Autodesk Inventor part; units mm, degrees
ref_plane "YZ Plane" through (0, 0, 0) normal (1, 0, 0) x (0, 1, 0)
ref_plane "XZ Plane" through (0, 0, 0) normal (0, 1, 0) x (-1, 0, 0)
ref_plane "XY Plane" through (0, 0, 0) normal (0, 0, 1) x (1, 0, 0)
sketch "Sketch1" plane through (0, 0, 0) normal (1, 0, 0) x (0, 1, 0)
  line L0 (7.987, -6.35) -> (11, -6.35)
  line L1 (11, -6.35) -> (11, -4.75)
  line L2 (11, -4.75) -> (8.75, -4.75)
  line L3 (8.75, -4.75) -> (8.75, 4.75)
  line L4 (8.75, 4.75) -> (11, 4.75)
  line L5 (11, 4.75) -> (11, 6.35)
  line L6 (11, 6.35) -> (7.987, 6.35)
  line L7 (7.987, 6.35) -> (7.987, 1.55)
  line L8 (7.987, 1.55) -> (6.945, 1.55)
  line L9 (6.945, 1.55) -> (6.945, -1.55)
  line L10 (6.945, -1.55) -> (7.987, -1.55)
  line L11 (7.987, -1.55) -> (7.987, -6.35)
  line L12 (0, 0) -> (0, 23.3621) construction
  line L13 (6.945, 0) -> (8.75, 0) construction
  dimension "d0" = 9.5
  dimension "d1" = 15.974
  dimension "d2" = 13.89
  dimension "d3" = 3.1
  dimension "d4" = 12.7
  dimension "d5" = 17.5
  dimension "d6" = 22
revolve "Revolution1" add sketch "Sketch1" angle 360 about axis through (0, 0, 0) along (0, 0, 1)
chamfer "Chamfer1" distance 0.3 angle 45 2 edges at (0, -7.987, 6.35) (0, -7.987, -6.35)
ref_plane "Work Plane1" through (0, 0, 0) normal (0, 0, -1) x (-1, 0, 0)
properties part number "idler pulley" material "ABS Plastic"
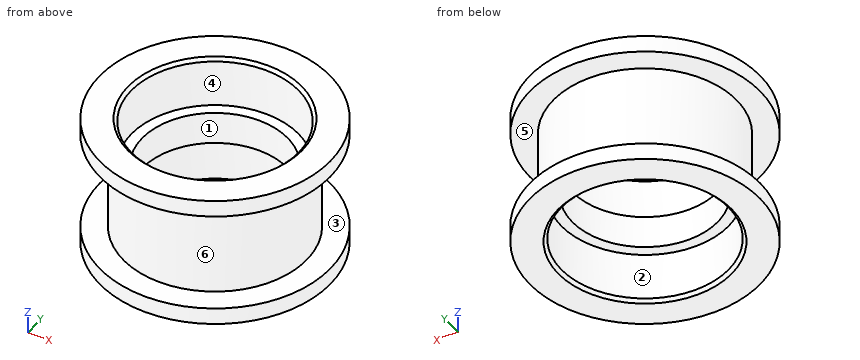
Source: CAD feature listing. Evaluate the final solid. Frame: model axes, mm. Face numbers are marked on the shaded views. A direction names the side the tool comes from. Give positions to 0.01 mm unless a question says otherwise; leave off trailing zeros. Loops run counter-clockwise (first coordinate to the right, second up) from the corner with the lowest first, then second, coordinate; pieces in that order, holes last. Notation, with made-up numbers: (65, -10) -> (75, -10) arc R25 ccw to (75, 13) -> close; hole circle Ø3 at (51, 10). An arc over 180 degrees is marked (long way). Use a Markdown table: item, result. Add a question column.
(1) Section query C-C (z = -3.5). Output: boundary loops of the cut face in (x, y), then the cut area to 3 significant figures.
(2) Section query A-A (x = 0). Output: boundary loops of the cut face in (y, z) (3 decimals), then the cut area to 3 significant figures.
(3) First-contact query: pin 1 Ø3 at (x, z) = (-4.5, 2) entering from -Y; pin 2 Ø13 at (x, y) = (0.5, -0.5) entering from -Z; pin 3 Ø4 at (x, z) = (-2, 3) entering from -Y. Flat tips, straight axial feed; report the tip coordinate or a pass-through.
(4) Pull-direction query (X, two-part tool) for the marked faces 4, 5 and 6; classes: +X half, -X half, draft (parallel to the pull), parting line (faces both ways), or undercut.
(5) Section query D-D (z = -1.25). Output: boundary loops of the cut face in (x, y) (3 decimals), then the cut area to 3 significant figures.
(6) Ray query, line 1 (Z direction, x = -9, y = -2.75); line 2 (Y direction, x = 0, z = -0.6) (3 decimals); line 3 (X direction, y = 0, z = -4.95). Return the intervals inside material, ascending.
(7) Access query for the marked faces 1, 2 and 3. Directions: +Z, -Z, +X, -X, +Y, -Y. A direction counts if a zero-diameter tool reaches every point of the face in a straight line with its end or side. Return the directions, or none.
Checked values:
| question | item | result |
|---|---|---|
| 1 | outline | circle Ø17.5 at (0, 0); hole circle Ø15.97 at (0, 0) |
| 1 | area | 40.1 mm^2 |
| 2 | outline | (-11, -6.35) -> (-8.287, -6.35) -> (-7.987, -6.05) -> (-7.987, -1.55) -> (-6.945, -1.55) -> (-6.945, 1.55) -> (-7.987, 1.55) -> (-7.987, 6.05) -> (-8.287, 6.35) -> (-11, 6.35) -> (-11, 4.75) -> (-8.75, 4.75) -> (-8.75, -4.75) -> (-11, -4.75) -> close; (6.945, -1.55) -> (7.987, -1.55) -> (7.987, -6.05) -> (8.287, -6.35) -> (11, -6.35) -> (11, -4.75) -> (8.75, -4.75) -> (8.75, 4.75) -> (11, 4.75) -> (11, 6.35) -> (8.287, 6.35) -> (7.987, 6.05) -> (7.987, 1.55) -> (6.945, 1.55) -> close |
| 2 | area | 40.1 mm^2 |
| 3 | pin 1 | y = -8.22 |
| 3 | pin 2 | z = -1.55 |
| 3 | pin 3 | y = -10.95 |
| 4 | face 4 | undercut |
| 4 | face 5 | draft |
| 4 | face 6 | parting line |
| 5 | outline | circle Ø17.5 at (0, 0); hole circle Ø13.89 at (0, 0) |
| 5 | area | 89.0 mm^2 |
| 6 | line 1 | -6.35 to -4.75, 4.75 to 6.35 |
| 6 | line 2 | -8.75 to -6.945, 6.945 to 8.75 |
| 6 | line 3 | -11 to -7.99, 7.99 to 11 |
| 7 | face 1 | +Z, -Z |
| 7 | face 2 | -Z |
| 7 | face 3 | none |
